```python
from build123d import *

# Parameters (mm, degrees)
SKETCH1_W               = 27.94
SKETCH1_H               = 25.9
BOSS_EXTRUDE1_DEPTH     = 5.08
SKETCH2_R               = 2.5
SKETCH2_R_2             = 1.25
BOSS_EXTRUDE2_DEPTH     = 11.4808
SKETCH3_R               = 1.25
CUT_EXTRUDE1_DEPTH      = 1
CUT_EXTRUDE1_DEPTH_BACK = 17.5608


with BuildPart() as part:
    # Sketch1 → Boss-Extrude1 (new body)
    with BuildSketch(Plane(origin=(0, 0, 0), x_dir=(1, 0, 0), z_dir=(0, 1, 0))):
        with Locations((2.687100719, -2.320830935)):
            Rectangle(SKETCH1_W, SKETCH1_H)
    extrude(amount=BOSS_EXTRUDE1_DEPTH)

    # Sketch2 → Boss-Extrude2 (add)
    with BuildSketch(Plane.XZ):
        with Locations((-9.082699611, 13.186946911)):
            Circle(SKETCH2_R)
        with Locations((-9.082699611, 13.186946911)):
            Circle(SKETCH2_R_2, mode=Mode.SUBTRACT)
        with Locations((13.624900389, 13.186946911)):
            Circle(SKETCH2_R)
        with Locations((13.624900389, 13.186946911)):
            Circle(SKETCH2_R_2, mode=Mode.SUBTRACT)
        with Locations((-9.082699611, -8.403053089)):
            Circle(SKETCH2_R)
        with Locations((-9.082699611, -8.403053089)):
            Circle(SKETCH2_R_2, mode=Mode.SUBTRACT)
        with Locations((13.624900389, -8.403053089)):
            Circle(SKETCH2_R)
        with Locations((13.624900389, -8.403053089)):
            Circle(SKETCH2_R_2, mode=Mode.SUBTRACT)
    extrude(amount=BOSS_EXTRUDE2_DEPTH)

    # Sketch3 → Cut-Extrude1 (cut, two sides)
    with BuildSketch(Plane(origin=(0, 5.08, 0), x_dir=(1, 0, 0), z_dir=(0, 1, 0))) as cut_extrude1_sk:
        with Locations((13.624900389, 8.403053089)):
            Circle(SKETCH3_R)
        with Locations((-9.082699611, 8.403053089)):
            Circle(SKETCH3_R)
        with Locations((13.624900389, -13.186946911)):
            Circle(SKETCH3_R)
        with Locations((-9.082699611, -13.186946911)):
            Circle(SKETCH3_R)
    extrude(amount=CUT_EXTRUDE1_DEPTH, mode=Mode.SUBTRACT)
    extrude(cut_extrude1_sk.sketch, amount=-CUT_EXTRUDE1_DEPTH_BACK, mode=Mode.SUBTRACT)


solid = part.part
```
Can you work these out from the model? Positions are in its coordinate system, mm. A direction names the side the tool comes from. Round coordinates to 2 decimals unless told otherwise and drop trailing zeros. Loops run counter-clockwise (first coordinate to the right, second up) from the corner with the lowest first, then second, coordinate; pieces in that order, holes last. Notation, with made-up numbers: M -22,83 L 2,83 A26 ccw 2,104 Z; hole C 13,-22.5 d3. An arc over 180 degrees is marked long. Answer as a JSON object with one key per item and string values. Group by question number.
Q1. Imagine slicing it at C-C, the plane y = -5.75. Please give me the cut outline in (x, z), then the cut area to 3 significant figures.
Q2. Imagine slicing it at D-D, the plane y = 3. Please give me the cut outline in (x, z), then the cut area to 3 significant figures.
Q3. Please list where these lines run through material, in increasing order: L1, parallel to Y at x = 12.5, z = 7.75; L2, parallel to X at y = 2.5, z = 4.5; L3, parallel to Z at x = -6, y = 0.75.
Q4. We'd pull the mould along Z, two halves only. Please class faces 1 (the flat face through (2, 5.08, 2)), 2 (the flat face through (2, 3, -10.629)), 3 (the flat face through (2, 0, 2)), 4 (the flat face through (2, 3, 15.271)): +Z half, -Z half, draft (parallel to the pull), parting line (faces both ways), or undercut.
Q5. Will these pins go through, and if not, where does the flat tip stop? pin 1 (1 mm diameter, centred on x = -2, z = 9.5, fed in from -Y); pin 2 (1.5 mm diameter, centred on y = 1.5, z = 8, fed in from -X); pin 3 (2 mm diameter, centred on x = -9.08, z = 13.19, fed in from +Y); pin 4 (4 mm diameter, centred on x = 5.5, y = 2, fed in from -Z).
Q6. On a 3-axis mill with a long thin cutter (end or side, diameter ignored), from which of +Z, -Z, +X, -X, +Y, -Y can I reach the whole of each face in a straight line? I mean faces 5 (the flat face through (-11.1, 0, 15)), 6 (the cylindrical face through (11.782, -5.66, 14.877)), 7 (the flat face through (-11.283, 3, 3)), 8 (the cylindrical face through (12.704, -3.084, 12.342)). Say none if no direction works.
Q7. Imagine slicing it at B-B, the plane x = -8.5. Please give me the cut outline in (y, z), then the cut area to 3 significant figures.
Q8. Imagine slicing it at A-A, the plane z = 12.5. Please give me the cut outline in (x, y), then the cut area to 3 significant figures.
Findings:
{
 "1": {"outline": "C -9.08,-8.4 d5; C -9.08,13.19 d5; C 13.62,-8.4 d5; C 13.62,13.19 d5; hole C -9.08,-8.4 d2.5; hole C -9.08,13.19 d2.5; hole C 13.62,-8.4 d2.5; hole C 13.62,13.19 d2.5", "area": "58.9 mm2"},
 "2": {"outline": "M -11.28,-10.63 L 16.66,-10.63 L 16.66,15.27 L -11.28,15.27 Z; hole C -9.08,-8.4 d2.5; hole C -9.08,13.19 d2.5; hole C 13.62,-8.4 d2.5; hole C 13.62,13.19 d2.5", "area": "704 mm2"},
 "3": {"L1": "y = 0 to 5.08", "L2": "x = -11.28 to 16.66", "L3": "z = -10.63 to 15.27"},
 "4": {"face 1": "draft", "face 2": "-Z half", "face 3": "undercut", "face 4": "+Z half"},
 "5": {"pin 1": "stops at y = 0", "pin 2": "stops at x = -11.28", "pin 3": "passes through", "pin 4": "stops at z = -10.63"},
 "6": {"face 5": "+Z, -X, -Y", "face 6": "-Y", "face 7": "+Z, -Z, -X, +Y", "face 8": "+Y, -Y"},
 "7": {"outline": "M -11.48,-10.83 L 0,-10.83 L 0,-10.63 L 5.08,-10.63 L 5.08,-9.51 L -11.48,-9.51 Z; M -11.48,-7.3 L 5.08,-7.3 L 5.08,12.08 L -11.48,12.08 L -11.48,10.76 L 0,10.76 L 0,-5.97 L -11.48,-5.97 Z; M -11.48,14.29 L 5.08,14.29 L 5.08,15.27 L 0,15.27 L 0,15.62 L -11.48,15.62 Z", "area": "170 mm2"},
 "8": {"outline": "M -11.49,-11.48 L -10.13,-11.48 L -10.13,5.08 L -11.28,5.08 L -11.28,0 L -11.49,0 Z; M -8.04,-11.48 L -6.68,-11.48 L -6.68,0 L 11.22,0 L 11.22,-11.48 L 12.58,-11.48 L 12.58,5.08 L -8.04,5.08 Z; M 14.67,-11.48 L 16.03,-11.48 L 16.03,0 L 16.66,0 L 16.66,5.08 L 14.67,5.08 Z", "area": "183 mm2"}
}
